```python
from build123d import *

# Parameters (mm, degrees)
SKETCH1_W           = 1.778
SKETCH1_H           = 6.35
BOSS_EXTRUDE1_DEPTH = 8.128
SKETCH2_R           = 2.032
CUT_EXTRUDE1_DEPTH  = 11.466526071


with BuildPart() as part:
    # Sketch1 → Boss-Extrude1 (new body)
    with BuildSketch(Plane.XY):
        with Locations((0.889, -3.175)):
            Rectangle(SKETCH1_W, SKETCH1_H)
    extrude(amount=BOSS_EXTRUDE1_DEPTH)

    # Sketch2 → Cut-Extrude1 (cut, through all)
    with BuildSketch(Plane.ZY):
        with Locations(Location((4.064, -3.175, 0), (0, 0, 270))):
            Circle(SKETCH2_R)
    extrude(amount=-CUT_EXTRUDE1_DEPTH, mode=Mode.SUBTRACT)


solid = part.part
```
Part model, mm, in its own coordinate system. Round coordinates to 2 decimals unless told otherwise and drop trailing zeros. Loops run counter-clockwise (first coordinate to the right, second up) from the corner with the lowest first, then second, coordinate; pieces in that order, holes last.
Item 1: Drop a flat-ended pin along its axis: P1, Ø3.5, axis at y = -3.175, z = 4.064, coming from the -X side. Give the stop position or say it passes through.
Item 2: Cut at B-B, the plane z = 5.5. Give the cut face in (x, y), then the cut area to 3 significant figures.
Item 3: Cut at A-A, the plane y = -4.25. Give the cut face in (x, z).
Item 4: Cut at C-C, the plane x = 0.95. Give the cut face in (y, z) (3 decimals), then the cut area to 3 significant figures.
Item 5: Mould opens along Z. For faces 1 (the face through (0.877, -5.113, 4.674)), 2 (the face through (1, -3, 8.128)), 3 (the face through (0, -2, 6)) say: +Z half, -Z half, draft (parallel to the pull), parting line (faces both ways), or undercut.
Item 6: Drill centre lines: line 1 (Y direction, x = 0.35, z = 4); line 2 (Z direction, x = 1.2, y = -3); line 3 (Z direction, x = 1.3, y = -2.5). Where is each one in solid material? Low to high.
A:
1. P1: passes through
2. outline: (0, -6.35) - (1.78, -6.35) - (1.78, -4.61) - (0, -4.61) - close; (0, -1.74) - (1.78, -1.74) - (1.78, 0) - (0, 0) - close
2. area: 6.18 mm2
3. outline: (0, 0) - (1.78, 0) - (1.78, 2.34) - (0, 2.34) - close; (0, 5.79) - (1.78, 5.79) - (1.78, 8.13) - (0, 8.13) - close
4. outline: (-6.35, 0) - (0, 0) - (0, 8.128) - (-6.35, 8.128) - close; hole circle Ø4.064 at (-3.175, 4.064)
4. area: 38.6 mm2
5. face 1: undercut
5. face 2: +Z half
5. face 3: draft
6. line 1: y = -6.35 to -5.21, -1.14 to 0
6. line 2: z = 0 to 2.04, 6.09 to 8.13
6. line 3: z = 0 to 2.15, 5.98 to 8.13
